Could you check a few things on this model? Use its own coordinates, in mm. Face numbers are marked on the shaded views. A direction names the side the tool comes from. Round coordinates to 2 decimals unless told otherwise and drop trailing zeros. Write each loop counter-clockwise with the first axis right and the second up, starting at its lowest first coordinate (ties: lowest second). Pieces come first, ordered by that corner, then holes. Notation, with made-up numbers: (4.25, 63.25) -> (47.25, 63.25) arc R18 ccw to (47.25, 90.25) -> close; hole circle Ø6 at (28.25, -29). An arc over 180 degrees is marked (long way). Answer in a Markdown table with one row per item.
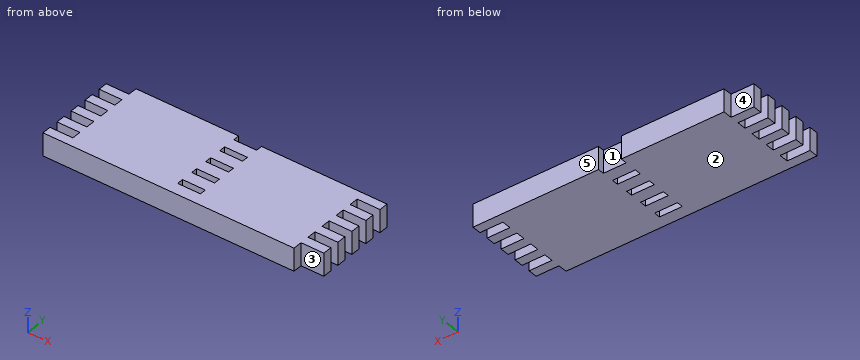
from build123d import *

# Parameters (mm, degrees)
SKETCH1_W           = 60
SKETCH1_H           = 20
BOSS_EXTRUDE1_DEPTH = 2.5
SKETCH2_W           = 5
SKETCH2_H           = 2
CUT_EXTRUDE1_DEPTH  = 33.015621187
SKETCH3_W           = 5
SKETCH3_H           = 2
CUT_EXTRUDE2_DEPTH  = 5
SKETCH4_W           = 5
SKETCH4_H           = 1.394303276
CUT_EXTRUDE3_DEPTH  = 5


with BuildPart() as part:
    # Sketch1 → Boss-Extrude1 (new, symmetric)
    with BuildSketch(Plane.XY):
        Rectangle(SKETCH1_W, SKETCH1_H)
    extrude(amount=BOSS_EXTRUDE1_DEPTH, both=True)

    # Sketch2 → Cut-Extrude1 (cut, through all)
    with BuildSketch(Plane.XY.offset(2.5)):
        with Locations((-27.5, 5)):
            Rectangle(SKETCH2_W, SKETCH2_H)
        with Locations((-27.5, 9)):
            Rectangle(SKETCH2_W, SKETCH2_H)
        with Locations((-27.5, 1)):
            Rectangle(SKETCH2_W, SKETCH2_H)
        with Locations((-27.5, -3)):
            Rectangle(SKETCH2_W, SKETCH2_H)
        with Locations((-27.5, -7)):
            Rectangle(SKETCH2_W, SKETCH2_H)
    extrude(amount=-CUT_EXTRUDE1_DEPTH, mode=Mode.SUBTRACT)

    # Sketch3 → Cut-Extrude2 (cut)
    with BuildSketch(Plane.XY.offset(2.5)):
        with Locations((27.5, -9)):
            Rectangle(SKETCH3_W, SKETCH3_H)
        with Locations((27.5, -5)):
            Rectangle(SKETCH3_W, SKETCH3_H)
        with Locations((27.5, -1)):
            Rectangle(SKETCH3_W, SKETCH3_H)
        with Locations((27.5, 3)):
            Rectangle(SKETCH3_W, SKETCH3_H)
        with Locations((27.5, 7)):
            Rectangle(SKETCH3_W, SKETCH3_H)
    extrude(amount=-CUT_EXTRUDE2_DEPTH, mode=Mode.SUBTRACT)

    # Sketch4 → Cut-Extrude3 (cut)
    with BuildSketch(Plane.XY.offset(2.5)):
        with Locations((0, 9.302848362)):
            Rectangle(SKETCH4_W, SKETCH4_H)
        with Locations((0, 5.302848362)):
            Rectangle(SKETCH4_W, SKETCH4_H)
        with Locations((0, 1.302848362)):
            Rectangle(SKETCH4_W, SKETCH4_H)
        with Locations((0, -2.697151638)):
            Rectangle(SKETCH4_W, SKETCH4_H)
        with Locations((0, -6.697151638)):
            Rectangle(SKETCH4_W, SKETCH4_H)
    extrude(amount=-CUT_EXTRUDE3_DEPTH, mode=Mode.SUBTRACT)


solid = part.part
1) Please list where these lines run through material, in increasing order: line 1 (Y direction, x = 0.5, z = 0.65); line 2 (Y direction, x = -27.5, z = -1.85); line 3 (X direction, y = -6.75, z = 1.35).
Findings:
| item | result |
|---|---|
| line 1 | y = -10 to -7.39, -6 to -3.39, -2 to 0.61, 2 to 4.61, 6 to 8.61 |
| line 2 | y = -10 to -8, -6 to -4, -2 to 0, 2 to 4, 6 to 8 |
| line 3 | x = -25 to -2.5, 2.5 to 30 |
2) Imagine slicing it at A-A, the plane x = 1. Please give me the cut outline in (y, z), plus the area to 3 significant figures.
Findings:
| item | result |
|---|---|
| outline | (-10, -2.5) -> (-7.39, -2.5) -> (-7.39, 2.5) -> (-10, 2.5) -> close; (-6, -2.5) -> (-3.39, -2.5) -> (-3.39, 2.5) -> (-6, 2.5) -> close; (-2, -2.5) -> (0.61, -2.5) -> (0.61, 2.5) -> (-2, 2.5) -> close; (2, -2.5) -> (4.61, -2.5) -> (4.61, 2.5) -> (2, 2.5) -> close; (6, -2.5) -> (8.61, -2.5) -> (8.61, 2.5) -> (6, 2.5) -> close |
| area | 65.1 mm^2 |
3) Thinking about a two-plate mould opening in X: for the marked faces 1 and 2, which applies, +X half, -X half, draft (parallel to the pull), parting line (faces both ways), or undercut?
Findings:
| item | result |
|---|---|
| face 1 | undercut |
| face 2 | draft |
4) For the marked faces 3, 4 and 5, which set-ups out of +Z, -Z, +X, -X, +Y, -Y let a thin tool reach every point of the face, with its end or its side?
Findings:
| item | result |
|---|---|
| face 3 | +Z, -Z, +X, -Y |
| face 4 | +Z, -Z, -X, +Y |
| face 5 | +Z, -Z, +X, -X, +Y |
5) For pin 1 (2.5 mm diameter, centred on x = -0.5, z = 0, fed in from +Y); pin 2 (1.6 mm diameter, centred on y = 9, z = -1, fed in from -X); pin 3 (2.5 mm diameter, centred on x = 28.5, z = 1, fed in from -Y), each with a flat end and sliding along its axis, tell me the tip position at first contact or that it passes through.
Findings:
| item | result |
|---|---|
| pin 1 | stops at y = 8.61 |
| pin 2 | stops at x = -25 |
| pin 3 | stops at y = -8 |
6) Imagine slicing it at B-B, the plane z = -0.6. Count the separate pieces of the cut face and the enclosed holes in it, plus the area to 3 significant figures.
Findings:
| item | result |
|---|---|
| separate pieces | 1 |
| enclosed holes | 4 |
| area | 1,070 mm^2 |
7) Imagine slicing it at C-C, the plane y = -5. Please give me the cut outline in (x, z), plus the area to 3 significant figures.
Findings:
| item | result |
|---|---|
| outline | (-30, -2.5) -> (25, -2.5) -> (25, 2.5) -> (-30, 2.5) -> close |
| area | 275 mm^2 |
